Verification items for the finished model (mm, model axes). A direction names the side the tool comes from. Give positions to 0.01 mm unless a question says otherwise; leave off trailing zeros. Write each loop counter-clockwise with the first axis right and the second up, starting at its lowest first coordinate (ties: lowest second). Pieces come first, ordered by that corner, then holes. Notation, with made-up numbers: (25, 35.25) - (39, 35.25) arc R20 cw to (39, 65.25) - close; hole circle Ø11 at (89.5, 69.25). An arc over 180 degrees is marked (long way). Put each result on its own line as item: value.
from build123d import *

# Parameters (mm, degrees)
F1_DEPTH  = 381
F3_W      = 1016
F3_H      = 457.2
F3_W_2    = 431.8
F3_H_2    = 355.6
F4_DEPTH  = 355.6
F5_DEPTH  = 1270
F6_W      = 63.5
F6_H      = 165.1
F7_DEPTH  = 25.4
F8_W      = 63.5
F8_H      = 165.1
F9_DEPTH  = 25.4
F10_W     = 63.5
F10_H     = 165.1
F11_DEPTH = 127
F12_W     = 127
F12_H     = 177.8
F13_DEPTH = 25.4
F14_W     = 1493.888004
F14_H     = 593.896151
F15_DEPTH = 355.601


with BuildPart() as f1:
    # F0 (on Top) → F1 (new body)
    with BuildSketch(Plane.XY):
        with BuildLine():
            Line((254, 1041.4), (-254, 1041.4))
            Line((-254, 1041.4), (-533.4, 787.4))
            Line((-533.4, 787.4), (-533.4, -914.4))
            ThreePointArc((-533.4, -914.4), (-496.202561, -1004.202561), (-406.4, -1041.4))
            Line((-406.4, -1041.4), (406.4, -1041.4))
            ThreePointArc((406.4, -1041.4), (496.202561, -1004.202561), (533.4, -914.4))
            Line((533.4, -914.4), (533.4, 787.4))
            Line((533.4, 787.4), (254, 1041.4))
        make_face()
    extrude(amount=F1_DEPTH)

    # F3 (on face) → F4 (cut)
    with BuildSketch(Plane.XY.offset(381)):
        with Locations((0, 254)):
            Rectangle(F3_W, F3_H)
        Polygon((-244.180185, 1016), (-508, 776.163805), (-508, 508), (508, 508), (508, 776.163805), (244.180185, 1016), align=None)
        with Locations((-292.1, -177.8)):
            Rectangle(F3_W_2, F3_H_2)
        with Locations((292.1, -177.8)):
            Rectangle(F3_W_2, F3_H_2)
        with Locations((292.1, -558.8)):
            Rectangle(F3_W_2, F3_H_2)
        with Locations((-292.1, -558.8)):
            Rectangle(F3_W_2, F3_H_2)
        with BuildLine():
            Line((50.8, 0), (-50.8, 0))
            Line((-50.8, 0), (-50.8, -381))
            Line((-50.8, -381), (-50.8, -762))
            Line((-50.8, -762), (-508, -762))
            Line((-508, -762), (-508, -914.4))
            ThreePointArc((-508, -914.4), (-478.242049, -986.242049), (-406.4, -1016))
            Line((-406.4, -1016), (406.4, -1016))
            ThreePointArc((406.4, -1016), (478.242049, -986.242049), (508, -914.4))
            Line((508, -914.4), (508, -762))
            Line((508, -762), (50.8, -762))
            Line((50.8, -762), (50.8, -381))
            Line((50.8, -381), (50.8, 0))
        make_face()
    extrude(amount=-F4_DEPTH, mode=Mode.SUBTRACT)

    # F2 (on Right) → F5 (cut, symmetric)
    with BuildSketch(Plane.YZ):
        Polygon((-1041.4, 381), (-1041.4, 228.6), (0, 228.6), (787.4, 381), align=None)
    extrude(amount=F5_DEPTH, both=True, mode=Mode.SUBTRACT)

    # F6 (on face) → F7 (cut, through all)
    with BuildSketch(Plane.XZ.offset(-482.6)):
        with Locations((0, 107.95)):
            Rectangle(F6_W, F6_H)
    extrude(amount=-F7_DEPTH, mode=Mode.SUBTRACT)

    # F8 (on face) → F9 (cut, through all)
    with BuildSketch(Plane.XZ):
        with Locations((0, 107.95)):
            Rectangle(F8_W, F8_H)
    extrude(amount=-F9_DEPTH, mode=Mode.SUBTRACT)

    # F10 (on Right) → F11 (cut, symmetric)
    with BuildSketch(Plane.YZ):
        with Locations((-82.55, 107.95)):
            Rectangle(F10_W, F10_H)
        with Locations((-463.55, 107.95)):
            Rectangle(F10_W, F10_H)
    extrude(amount=F11_DEPTH, both=True, mode=Mode.SUBTRACT)

    # F12 (on face) → F13 (cut)
    with BuildSketch(Plane(origin=(0, 1041.4, 0), x_dir=(-1, 0, 0), z_dir=(0, 1, 0))):
        with Locations((0, 114.3)):
            Rectangle(F12_W, F12_H)
        with BuildLine():
            Line((-63.5, 203.2), (63.5, 203.2))
            ThreePointArc((63.5, 203.2), (0, 266.7), (-63.5, 203.2))
        make_face()
    extrude(amount=-F13_DEPTH, mode=Mode.SUBTRACT)

    # F14 (on face) → F15 (cut, through all)
    with BuildSketch(Plane.XY.offset(25.4)):
        with Locations((0, 779.548075)):
            Rectangle(F14_W, F14_H)
    extrude(amount=F15_DEPTH, mode=Mode.SUBTRACT)


solid = f1.part
Q1. Section check D-D, the plane x = 445. Record the cut outline in (y, z), plus the area to 3 significant figures.
Answers follow:
outline: (-1035.39, 0) - (867.76, 0) - (867.76, 25.4) - (25.4, 25.4) - (25.4, 233.52) - (0, 228.6) - (0, 25.4) - (-355.6, 25.4) - (-355.6, 228.6) - (-381, 228.6) - (-381, 25.4) - (-736.6, 25.4) - (-736.6, 228.6) - (-762, 228.6) - (-762, 25.4) - (-1008.38, 25.4) - (-1008.38, 228.6) - (-1035.39, 228.6) - close
area: 69,400 mm2
Q2. Set-up check for faces 4 (the face through (82, -755, 228.6)), 5 (the face through (-295, -355.6, 128)), 6 (the face through (508, 251, 143)): record each of +Z, -Z, +X, -X, +Y, -Y from which the full face is reachable in a straight line by a thin tool's end or side.
Answers follow:
face 4: +Z, +X, -X, -Y
face 5: +Z
face 6: +Z, +Y
Q3. Scan lines: line 1 along Y through (x, z) = (-113, 45); line 2 along X through (y, z) = (-342, 187); line 3 along Y through (x, z) = (55, 53). Record each from-to range of solid material in increasing order.
Answers follow:
line 1: y = -1041.4 to -1016, -762 to -736.6, -381 to -355.6, 0 to 25.4
line 2: x = -533.4 to -508, -76.2 to -50.8, 50.8 to 76.2, 508 to 533.4
line 3: y = -1041.4 to -1016, -762 to -495.3, -431.8 to -114.3, -50.8 to 25.4
Q4. Section check A-A, the plane x = -146. Record the cut outline in (y, z), plus the area to 3 significant figures.
Answers follow:
outline: (-1041.4, 0) - (1041.4, 0) - (1041.4, 25.4) - (25.4, 25.4) - (25.4, 233.52) - (0, 228.6) - (0, 25.4) - (-355.6, 25.4) - (-355.6, 228.6) - (-381, 228.6) - (-381, 25.4) - (-736.6, 25.4) - (-736.6, 228.6) - (-762, 228.6) - (-762, 25.4) - (-1016, 25.4) - (-1016, 228.6) - (-1041.4, 228.6) - close
area: 73,600 mm2
Q5. Release check for a two-part mould opening along X. For faces 1 (the face through (-391.74, 916.18, 12.52)), 2 (the face through (-508, -561, 128)), 3 (the face through (-6, -1041.4, 113)) record: released by +X, released by -X, zero draft, split by the parting line, or undercut.
Answers follow:
face 1: released by -X
face 2: undercut
face 3: zero draft
Q6. Section check C-C, the plane y = 420. Record the cut outline in (x, z), plus the area to 3 significant figures.
Answers follow:
outline: (-533.4, 0) - (533.4, 0) - (533.4, 309.89) - (508, 309.89) - (508, 25.4) - (-508, 25.4) - (-508, 309.89) - (-533.4, 309.89) - close
area: 41,500 mm2
Q7. Section check B-B, the plane y = -238. Record the cut outline in (x, z).
Answers follow:
outline: (-533.4, 0) - (533.4, 0) - (533.4, 228.6) - (508, 228.6) - (508, 25.4) - (76.2, 25.4) - (76.2, 228.6) - (50.8, 228.6) - (50.8, 25.4) - (-50.8, 25.4) - (-50.8, 228.6) - (-76.2, 228.6) - (-76.2, 25.4) - (-508, 25.4) - (-508, 228.6) - (-533.4, 228.6) - close
Q8. Go/stop test with flat-tipped pins: pin 1 Ø20.5 at (x, z) = (61, 140) entering from +Y; pin 2 Ø4 at (x, y) = (-233.5, 281) entering from +Z. Record where each tip stops, or that it passes through.
Answers follow:
pin 1: stops at y = 25.4
pin 2: stops at z = 25.4
